CAD build for the part. Positions are in the model's coordinates, mm. Face numbers are marked on the shaded views. A direction names the side the tool comes from. Coordinates: 2 decimals unless noted, no trailing zeros. Loops run counter-clockwise (first coordinate to the right, second up) from the corner with the lowest first, then second, coordinate; pieces in that order, holes last. Notation, with made-up numbers: (42.5, -19) -> (71.5, -19) arc R18 ccw to (71.5, 4) -> close; hole circle Ø2 at (55, 41.25). An arc over 180 degrees is marked (long way). Write each question's results on one line, items separated by ' | '.
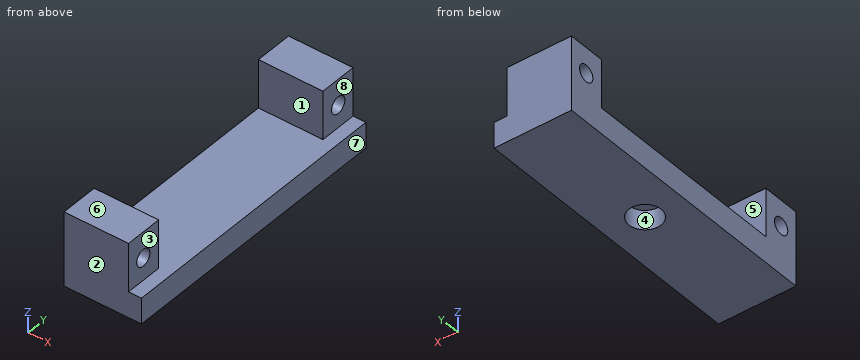
```python
from build123d import *

# Parameters (mm, degrees)
F1_DEPTH = 7.62
F3_R     = 1.651
F4_DEPTH = 25.4
F5_R     = 3.175
F6_DEPTH = 3.81
F7_W     = 55.88
F7_H     = 9.525
F8_DEPTH = 2.54


with BuildPart() as f1:
    # F0 (on Right) → F1 (new body, symmetric)
    with BuildSketch(Plane.YZ):
        Polygon((0, 0), (0, -5.08), (27.94, -5.08), (27.94, 9.525), (20.447, 9.525), (20.447, 0), align=None)
    extrude(amount=F1_DEPTH, both=True)

    # F2: F1 across plane


with BuildPart() as f1_1:
    add(f1.part)
    add(f1.part.mirror(Plane.XZ))

    # F3 (on face) → F4 (cut)
    with BuildSketch(Plane.YZ.offset(7.62)):
        with Locations((-24.257, 4.445)):
            Circle(F3_R)
        with Locations((24.257, 4.445)):
            Circle(F3_R)
    extrude(amount=-F4_DEPTH, mode=Mode.SUBTRACT)

    # F5 (on face) → F6 (cut)
    with BuildSketch(Plane(origin=(0, 0, -5.08), x_dir=(1, 0, 0), z_dir=(0, 0, -1))):
        Circle(F5_R)
    extrude(amount=-F6_DEPTH, mode=Mode.SUBTRACT)

    # F7 (on face) → F8 (cut)
    with BuildSketch(Plane.YZ.offset(7.62)):
        with Locations((0, 4.7625)):
            Rectangle(F7_W, F7_H)
    extrude(amount=-F8_DEPTH, mode=Mode.SUBTRACT)


solid = f1_1.part
```
Q1. Cut at D-D on x = 6. Write the cut outline in (y, z).
Results are:
outline: (-27.94, -5.08) -> (27.94, -5.08) -> (27.94, 0) -> (-27.94, 0) -> close
Q2. Cut at A-A on z = 8.75. Write the cut outline in (x, y).
Results are:
outline: (-7.62, -27.94) -> (5.08, -27.94) -> (5.08, -20.45) -> (-7.62, -20.45) -> close; (-7.62, 20.45) -> (5.08, 20.45) -> (5.08, 27.94) -> (-7.62, 27.94) -> close
Q3. Pull direction Y, two halves, no side cores. Call the marked faces 1, 2 and 3: +Y half, -Y half, draft (parallel to the pull), parting line (faces both ways), or undercut.
Results are:
face 1: undercut | face 2: -Y half | face 3: draft
Q4. Drop flat-ended pins along their axis: pin 1 (4.5 mm diameter, centred on y = 24.257, z = 4.445, fed in from +X); pin 2 (5 mm diameter, centred on x = 1, y = -0.5, fed in from -Z). Give the stop position or say it passes through.
Results are:
pin 1: x = 5.08 | pin 2: z = -5.08
Q5. Cut at C-C on y = -1. Write the cut outline in (x, z), and give its area (3 significant figures).
Results are:
outline: (-7.62, -5.08) -> (-3.01, -5.08) -> (-3.01, -1.27) -> (3.01, -1.27) -> (3.01, -5.08) -> (7.62, -5.08) -> (7.62, 0) -> (-7.62, 0) -> close | area: 54.5 mm^2
Q6. Cut at B-B on x = 0.75. Write the cut outline in (y, z) (3 decimals), and give its area (3 significant figures).
Results are:
outline: (-27.94, -5.08) -> (-3.085, -5.08) -> (-3.085, -1.27) -> (3.085, -1.27) -> (3.085, -5.08) -> (27.94, -5.08) -> (27.94, 9.525) -> (20.447, 9.525) -> (20.447, 0) -> (-20.447, 0) -> (-20.447, 9.525) -> (-27.94, 9.525) -> close; hole circle Ø3.302 at (-24.257, 4.445); hole circle Ø3.302 at (24.257, 4.445) | area: 386 mm^2
Q7. Wall check: L1, parallel to Y at x = -4.25, z = 6.5; L2, parallel to X at y = 0, z = -2.4 (3 decimals); L3, parallel to Z at x = 0.5, y = 8. Give the ranges that are in metal, low to high. Write a range as from..to.
Results are:
L1: -27.94..-20.45, 20.45..27.94 | L2: -7.62..-3.175, 3.175..7.62 | L3: -5.08..0
Q8. Which spindle directions (+Z, -Z, +X, -X, +Y, -Y) get a long thin tool onto all of the face, cutting with end or side? Do the marked faces 4, 5, 6, 7 and 8. Say none if no direction does.
Results are:
face 4: -Z | face 5: +Z, +X, -X | face 6: +Z, +X, -X, +Y, -Y | face 7: +Z, -Z, +X, +Y, -Y | face 8: +Z, +X, +Y, -Y
